The drawing under review shows one solid part. Ordinate dimensions are in mm from its lowest x, y, z. A direction names the side the tool comes from. Give positions to 0.01 mm unless a question says otherwise; leave off trailing zeros. Write each loop counter-clockwise with the first axis right and the second up, starting at its lowest first coordinate (ties: lowest second). Pieces come first, ordered by that corner, then holes.
Q1. Insertion check: P1, Ø6, axis at y = 11.5, z = 44, coming from the +X side; P2, Ø3, axis at x = 118.5, y = 8.5, coming from the -Z side; P3, Ø6, axis at y = 15, z = 90.5, coming from the +X side. Each pin has a flat end and moves straight along its axis. Give the tip position at first contact, or say it passes through.
Q2. We need section C-C (z = 27). Write out the cut boundary in (x, y).
Q3. For line 1 (Y direction, x = 42.75, z = 105.5); line 2 (X direction, y = 11.25, z = 45.5); line 3 (X direction, y = 9.25, z = 110.5), list the stretches that pass through material, from the lowest coordinate up.
Q4. We need section D-D (x = 124). Write out the cut boundary in (y, z).
Q5. We need section B-B (y = 16.25). Write out the cut boundary in (x, z), then the cut area to 4 significant figures.
Q6. Machinability: for the marked faces 1 and 2, which of the approach directions +Z, -Z, +X, -X, +Y, -Y give a long, thin tool a straight path to every point of the face, cutting with its end or side? Answer none if there is none.
Q7. We need section A-A (x = 42.75). Write out the cut boundary in (y, z), then the cut area to 3 significant figures.
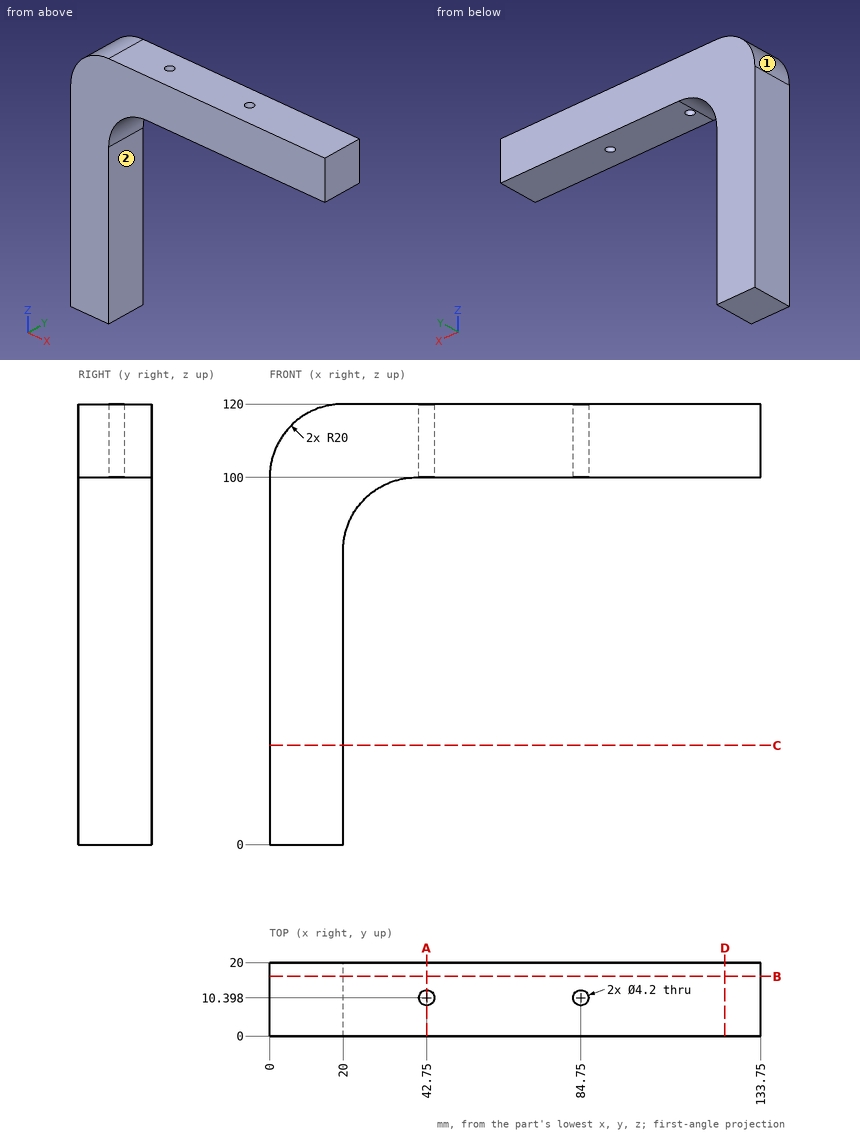
Computed:
1. P1: stops at x = 20
1. P2: stops at z = 100
1. P3: stops at x = 25.24
2. outline: (0, 0) - (20, 0) - (20, 20) - (0, 20) - close
3. line 1: y = 0 to 8.3, 12.5 to 20
3. line 2: x = 0 to 20
3. line 3: x = 2.98 to 40.99, 44.51 to 82.99, 86.51 to 133.75
4. outline: (0, 100) - (20, 100) - (20, 120) - (0, 120) - close
5. outline: (0, 0) - (20, 0) - (20, 80) arc R20 cw to (40, 100) - (133.75, 100) - (133.75, 120) - (20, 120) arc R20 ccw to (0, 100) - close
5. area: 4,675 mm2
6. face 1: +Z, -X, +Y, -Y
6. face 2: -Z, +X, +Y, -Y
7. outline: (0, 100) - (8.3, 100) - (8.3, 120) - (0, 120) - close; (12.5, 100) - (20, 100) - (20, 120) - (12.5, 120) - close
7. area: 316 mm2
